```python
from build123d import *

# Parameters (mm, degrees)
SKETCH_1_R      = 10
EXTRUDE_1_DEPTH = 150
SKETCH_2_W      = 35
SKETCH_2_H      = 20
EXTRUDE_2_DEPTH = 35
SKETCH_3_W      = 6
SKETCH_3_H      = 6
SKETCH_3_R      = 0.5
EXTRUDE_3_DEPTH = 15


with BuildPart() as part:
    # 草图1 → 凸台-拉伸1 (new, symmetric)
    with BuildSketch(Plane(origin=(0, 0, 0), x_dir=(0, 0, -1), z_dir=(1, 0, 0))):
        Circle(SKETCH_1_R)
    extrude(amount=EXTRUDE_1_DEPTH, both=True)

    # 草图2 → 凸台-拉伸2 (add)
    with BuildSketch(Plane.XY):
        with Locations((132.5, 0)):
            Rectangle(SKETCH_2_W, SKETCH_2_H)
    extrude(amount=EXTRUDE_2_DEPTH)

    # 草图3 → 凸台-拉伸3 (add)
    # profile 1 of 2: a face of its own
    with BuildSketch(Plane.XY.offset(35)):
        with Locations((141.458586474, 0)):
            Rectangle(SKETCH_3_W, SKETCH_3_H)
        with Locations((141.458586474, 0)):
            Circle(SKETCH_3_R, mode=Mode.SUBTRACT)
    # profile 2 of 2: a face of its own
    with BuildSketch(Plane.XY.offset(35)):
        with Locations((141.458586474, 0)):
            Circle(SKETCH_3_R)
    extrude(amount=EXTRUDE_3_DEPTH)


solid = part.part
```
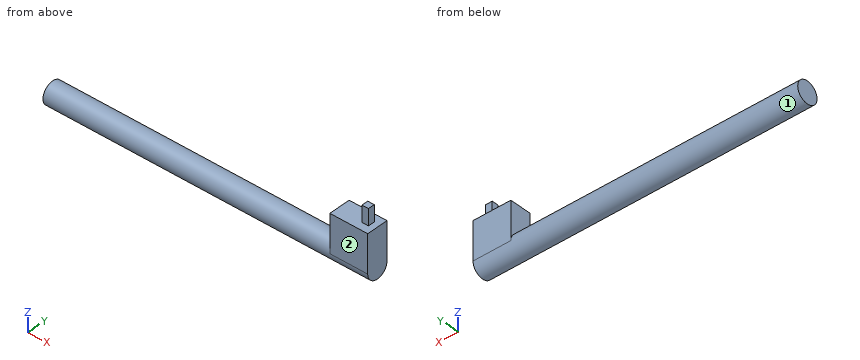
Verification items for the finished model (mm, model axes). Face numbers are marked on the shaded views. A direction names the side the tool comes from. Give positions to 0.01 mm unless a question says otherwise; leave off trailing zeros. Order: outer loops, then holes, each group sorted by start corner. A loop starts at its lowest first (then second) coordinate and runs counter-clockwise, first axis right, second up. Notation, with made-up numbers: (43.5, 30.25) -> (88.5, 30.25) arc R32 cw to (88.5, 67.25) -> close; hole circle Ø5 at (42, -9). An arc over 180 degrees is marked (long way). One line per item, written item: value.
(1) Sectioned sample at C-C on z = 42. Record the cut outline in (x, y), then the cut area to 3 significant figures.
Final values:
outline: (138.46, -3) -> (144.46, -3) -> (144.46, 3) -> (138.46, 3) -> close
area: 36.0 mm^2
(2) Scan lines: line 1 along X through (y, z) = (3.5, 19); line 2 along Z through (x, y) = (-103.5, 0); line 3 along Y through (x, z) = (85, -1). Record each from-to range of solid material in increasing order. Write a range as [from, to].
Final values:
line 1: [115, 150]
line 2: [-10, 10]
line 3: [-9.95, 9.95]
(3) Gauge pin test, flat ends, axial feed: pin 1 (1 mm diameter, centred on x = -111.5, y = 1, fed in from -Z); pin 2 (5 mm diameter, centred on x = 141.5, z = 44.5, fed in from +Y); pin 3 (5 mm diameter, centred on x = 140, z = 41, fed in from -Y). Record the tip position at first contact, or that the pin passes through.
Final values:
pin 1: z = -9.99
pin 2: y = 3
pin 3: y = -3
(4) Sectioned sample at D-D on z = 3. Record the cut outline in (x, y), then the cut area to 3 significant figures.
Final values:
outline: (-150, -9.54) -> (115, -9.54) -> (115, -10) -> (150, -10) -> (150, 10) -> (115, 10) -> (115, 9.54) -> (-150, 9.54) -> close
area: 5,760 mm^2
(5) Sectioned sample at B-B on x = -69. Record the cut outline in (y, z).
Final values:
outline: circle Ø20 at (0, 0)
(6) Sectioned sample at A-A on y = 6. Record the cut outline in (x, z), then the cut area to 4 significant figures.
Final values:
outline: (-150, -8) -> (150, -8) -> (150, 35) -> (115, 35) -> (115, 8) -> (-150, 8) -> close
area: 5,745 mm^2
(7) Tool access check on the marked faces 1 and 2. Record the directions out of +Z, -Z, +X, -X, +Y, -Y that give a thin tool (end or side, any length) a straight path to the whole face; none if there is none.
Final values:
face 1: -X
face 2: +Z, -Z, +X, -X, -Y
